from build123d import *

# Parameters (mm, degrees)
BOSS_EXTRUDE1_DEPTH = 1.6
SKETCH2_R           = 1.016
CUT_EXTRUDE1_DEPTH  = 44.666207109
SKETCH3_R           = 0.3048
CUT_EXTRUDE2_DEPTH  = 44.666207109
CUT_EXTRUDE3_DEPTH  = 44.666207109


with BuildPart() as part:
    # Sketch6 → Boss-Extrude1 (new body)
    with BuildSketch(Plane(origin=(0, 3.4925, 0), x_dir=(1, 0, 0), z_dir=(0, 1, 0))):
        with BuildLine():
            Line((14.097, 17.653), (14.097, 32.9565))
            ThreePointArc((14.097, 32.9565), (13.278656347, 34.932156347), (11.303, 35.7505))
            Line((11.303, 35.7505), (5.9055, 35.7505))
            ThreePointArc((5.9055, 35.7505), (5.680993597, 35.843493597), (5.588, 36.068))
            Line((5.588, 36.068), (5.588, 37.084))
            ThreePointArc((5.588, 37.084), (5.495006403, 37.308506403), (5.2705, 37.4015))
            Line((5.2705, 37.4015), (-5.2705, 37.4015))
            ThreePointArc((-5.2705, 37.4015), (-5.495006403, 37.308506403), (-5.588, 37.084))
            Line((-5.588, 37.084), (-5.588, 36.068))
            ThreePointArc((-5.588, 36.068), (-5.680993597, 35.843493597), (-5.9055, 35.7505))
            Line((-5.9055, 35.7505), (-11.303, 35.7505))
            ThreePointArc((-11.303, 35.7505), (-13.278656347, 34.932156347), (-14.097, 32.9565))
            Line((-14.097, 32.9565), (-14.097, 17.653))
            ThreePointArc((-14.097, 17.653), (-14.39457951, 16.93457951), (-15.113, 16.637))
            Line((-15.113, 16.637), (-19.685, 16.637))
            ThreePointArc((-19.685, 16.637), (-21.660656347, 15.818656347), (-22.479, 13.843))
            Line((-22.479, 13.843), (-22.479, -10.16))
            ThreePointArc((-22.479, -10.16), (-21.660656347, -12.135656347), (-19.685, -12.954))
            Line((-19.685, -12.954), (-15.113, -12.954))
            ThreePointArc((-15.113, -12.954), (-14.39457951, -13.25157951), (-14.097, -13.97))
            Line((-14.097, -13.97), (-14.097, -17.653))
            Line((-14.097, -17.653), (-14.097, -23.622))
            ThreePointArc((-14.097, -23.622), (-13.278656347, -25.597656347), (-11.303, -26.416))
            Line((-11.303, -26.416), (11.303, -26.416))
            ThreePointArc((11.303, -26.416), (13.278656347, -25.597656347), (14.097, -23.622))
            Line((14.097, -23.622), (14.097, -17.653))
            Line((14.097, -17.653), (14.097, -13.97))
            ThreePointArc((14.097, -13.97), (14.39457951, -13.25157951), (15.113, -12.954))
            Line((15.113, -12.954), (19.685, -12.954))
            ThreePointArc((19.685, -12.954), (21.660656347, -12.135656347), (22.479, -10.16))
            Line((22.479, -10.16), (22.479, 13.843))
            ThreePointArc((22.479, 13.843), (21.660656347, 15.818656347), (19.685, 16.637))
            Line((19.685, 16.637), (15.113, 16.637))
            ThreePointArc((15.113, 16.637), (14.39457951, 16.93457951), (14.097, 17.653))
        make_face()
    extrude(amount=BOSS_EXTRUDE1_DEPTH)

    # Sketch2 → Cut-Extrude1 (cut, through all)
    with BuildSketch(Plane(origin=(0, 3.4925, 0), x_dir=(1, 0, 0), z_dir=(0, 1, 0))):
        with Locations(Location((19.685, 13.843, 0), (0, 0, 90))):
            Circle(SKETCH2_R)
        with Locations(Location((19.685, -9.66, 0), (0, 0, 90))):
            Circle(SKETCH2_R)
        with Locations(Location((-19.685, -9.66, 0), (0, 0, 90))):
            Circle(SKETCH2_R)
        with Locations(Location((-19.685, 13.843, 0), (0, 0, 90))):
            Circle(SKETCH2_R)
    extrude(amount=CUT_EXTRUDE1_DEPTH, mode=Mode.SUBTRACT)

    # Sketch3 → Cut-Extrude2 (cut, through all)
    with BuildSketch(Plane(origin=(0, 3.4925, 0), x_dir=(1, 0, 0), z_dir=(0, 1, 0))):
        with Locations(Location((-4.445, 33.613, 0), (0, 0, 270))):
            Circle(SKETCH3_R)
        with Locations(Location((-3.175, 33.613, 0), (0, 0, 270))):
            Circle(SKETCH3_R)
        with Locations(Location((-1.905, 33.613, 0), (0, 0, 270))):
            Circle(SKETCH3_R)
        with Locations(Location((-0.635, 33.613, 0), (0, 0, 270))):
            Circle(SKETCH3_R)
        with Locations(Location((0.635, 33.613, 0), (0, 0, 270))):
            Circle(SKETCH3_R)
        with Locations(Location((1.905, 33.613, 0), (0, 0, 270))):
            Circle(SKETCH3_R)
        with Locations(Location((3.175, 33.613, 0), (0, 0, 270))):
            Circle(SKETCH3_R)
        with Locations(Location((4.445, 33.613, 0), (0, 0, 270))):
            Circle(SKETCH3_R)
        with Locations(Location((-3.175, 34.883, 0), (0, 0, 270))):
            Circle(SKETCH3_R)
        with Locations(Location((-1.905, 34.883, 0), (0, 0, 270))):
            Circle(SKETCH3_R)
        with Locations(Location((-0.635, 34.883, 0), (0, 0, 270))):
            Circle(SKETCH3_R)
        with Locations(Location((0.635, 34.883, 0), (0, 0, 270))):
            Circle(SKETCH3_R)
        with Locations(Location((1.905, 34.883, 0), (0, 0, 270))):
            Circle(SKETCH3_R)
        with Locations(Location((3.175, 34.883, 0), (0, 0, 270))):
            Circle(SKETCH3_R)
        with Locations(Location((4.445, 34.883, 0), (0, 0, 270))):
            Circle(SKETCH3_R)
        with Locations(Location((-4.445, 34.883, 0), (0, 0, 270))):
            Circle(SKETCH3_R)
    extrude(amount=CUT_EXTRUDE2_DEPTH, mode=Mode.SUBTRACT)

    # Sketch8 → Cut-Extrude3 (cut, through all)
    with BuildSketch(Plane.XZ.offset(-3.4925)):
        with BuildLine():
            Line((-12.64, -4.01), (3.86, -4.01))
            ThreePointArc((3.86, -4.01), (4.920660172, -4.449339828), (5.36, -5.51))
            Line((5.36, -5.51), (5.36, -6.51))
            ThreePointArc((5.36, -6.51), (4.920660172, -7.570660172), (3.86, -8.01))
            Line((3.86, -8.01), (-12.64, -8.01))
            ThreePointArc((-12.64, -8.01), (-13.700660172, -7.570660172), (-14.14, -6.51))
            Line((-14.14, -6.51), (-14.14, -5.51))
            ThreePointArc((-14.14, -5.51), (-13.700660172, -4.449339828), (-12.64, -4.01))
        make_face()
    extrude(amount=-CUT_EXTRUDE3_DEPTH, mode=Mode.SUBTRACT)


solid = part.part
Verification items for the finished model (mm, model axes). A direction names the side the tool comes from. Give positions to 0.01 mm unless a question says otherwise; leave off trailing zeros. Loops run counter-clockwise (first coordinate to the right, second up) from the corner with the lowest first, then second, coordinate; pieces in that order, holes last.
1. Tool access check on faces 5 (the flat face through (-9, 4, -35.75)), 6 (the flat face through (9, 4, -35.75)), 7 (the flat face through (-5, 4, -4.01)), 8 (the cylindrical face through (-13.3, 4.281, 25.576)). Record the directions out of +Z, -Z, +X, -X, +Y, -Y that give a thin tool (end or side, any length) a straight path to the whole face; none if there is none.
Derived:
face 5: -Z, -X, +Y, -Y
face 6: -Z, +X, +Y, -Y
face 7: +Y, -Y
face 8: +Z, -X, +Y, -Y
2. Cross-section at C-C on y = 4.6. Count the separate pieces of the cut face and the enclosed holes in it, and give its area (3 significant figures).
Derived:
separate pieces: 1
enclosed holes: 21
area: 2,160 mm2
3. Release check for a two-part mould opening along X. For faces 1 (the flat face through (0, 5.092, 1)), 2 (the cylindrical face through (4.93, 4.28, -7.56)), 3 (the cylindrical face through (4.91, 4.28, -4.44)), 4 (the cylindrical face through (-21.64, 4.28, -15.84)) record: +X half, -X half, draft (parallel to the pull), parting line (faces both ways), or undercut.
Derived:
face 1: draft
face 2: undercut
face 3: undercut
face 4: -X half
4. Cross-section at B-B on z = -25.5. Record the cut outline in (x, y).
Derived:
outline: (-14.1, 3.49) - (14.1, 3.49) - (14.1, 5.09) - (-14.1, 5.09) - close
5. Go/stop test with flat-tipped pins: P1, Ø0.8, axis at x = -17.5, y = 4, coming from the +Z side; P2, Ø0.8, axis at y = 4, z = 19.5, coming from the -X side; P3, Ø0.5, axis at y = 4, z = -22.5, coming from the +X side. Record where each tip stops, or that it passes through.
Derived:
P1: stops at z = 12.95
P2: stops at x = -14.1
P3: stops at x = 14.1
6. Cross-section at A-A on x = -12. Record the cut outline in (y, z).
Derived:
outline: (3.49, -35.66) - (5.09, -35.66) - (5.09, -8.01) - (3.49, -8.01) - close; (3.49, -4.01) - (5.09, -4.01) - (5.09, 26.33) - (3.49, 26.33) - close
7. Material ranges on probe 1 along X at (y, z) = (4.6, -6.5); probe 2 along X at (y, z) = (4.1, 21); probe 3 along Z at (x, y) = (9.5, 4.25), recorded low to high.
Derived:
probe 1: x = -22.48 to -14.14, 5.36 to 22.48
probe 2: x = -14.1 to 14.1
probe 3: z = -35.75 to 26.42
